Autodesk Inventor part; units mm, degrees
ref_plane "YZ Plane" through (0, 0, 0) normal (1, 0, 0) x (0, 1, 0)
ref_plane "XZ Plane" through (0, 0, 0) normal (0, 1, 0) x (-1, 0, 0)
ref_plane "XY Plane" through (0, 0, 0) normal (0, 0, 1) x (1, 0, 0)
sketch "Sketch1" plane through (0, 0, 0) normal (0, 1, 0) x (-1, 0, 0)
  circle A0 centre (0, 0) radius 14
  circle A1 centre (0, 0) radius 14
  dimension "d0" = 28
extrude "Extrusion1" add sketch "Sketch1" along normal blind 1
sketch "Sketch2" plane through (0, 1, 0) normal (0, 1, 0) x (1, 0, 0)
  circle A0 centre (0, 0) radius 13.25
  dimension "d4" = 26.5
extrude "Extrusion2" add sketch "Sketch2" along normal blind 3
sketch "Sketch3" plane through (0, 4, 0) normal (0, 1, 0) x (1, 0, 0)
  circle A0 centre (0, 0) radius 14
  dimension "d7" = 28
extrude "Extrusion3" add sketch "Sketch3" along normal blind 1
sketch "Sketch4" plane through (0, 5, 0) normal (0, 1, 0) x (1, 0, 0)
  circle A0 centre (0, 0) radius 1.25
  dimension "d10" = 2.5
hole "Hole1" at (0, 5, 0) direction (0, -1, 0) diameter 2.5 end through all
equation "\"d16\" = Thickness"
equation "\"BendRadius\" = Thickness"
equation "\"BendReliefWidth\" = Thickness"
equation "\"BendReliefDepth\" = 0.5 * Thickness"
equation "\"CornerReliefSize\" = 4 * Thickness"
equation "\"MinimumRemnant\" = 2 * Thickness"
equation "\"TransitionRadius\" = BendRadius"
equation "\"JacobiRadiusSize\" = BendRadius"
equation "\"GapSize\" = Thickness"
properties part number "wheeltemplate"
Source: CAD feature listing. Evaluate the final solid. Frame: model axes, mm. A direction names the side the tool comes from. Round coordinates to 2 decimals unless told otherwise and drop trailing zeros. Loops run counter-clockwise (first coordinate to the right, second up) from the corner with the lowest first, then second, coordinate; pieces in that order, holes last. Notation, with made-up numbers: (-31, 66.25) - (3, 66.25) arc R20 cw to (3, 79.25) - close; hole circle Ø8 at (9, -16.5). An arc over 180 degrees is marked (long way). Write item = value, one per line. Start each with the question number.
(1) Section query B-B, the plane z = 0. Output: boundary loops of the cut face in (x, y), plus the area to 3 significant figures.
(2) Section query D-D, the plane x = 11.5. Output: boundary loops of the cut face in (y, z), plus the area to 3 significant figures.
(3) Pin query (flat end, axial travel): pin 1 (1.5 mm diameter, centred on y = 3, z = -1, fed in from +X). Return the tip coordinate at first contact, or that it passes through.
(4) Ray query, line 1 along Z through (x, y) = (0, 1.3); line 2 along X through (y, z) = (4.4, -1). Return the intervals inside material, ascending. Write a range as from..to.
(5) Set-up query: faces 1 (the face through (-12.932, 0.493, 5.362)), 2 (the face through (-12.4, 1, -5.1)). Return all of +Z, -Z, +X, -X, +Y, -Y with unobstructed straight access to the full face (end or side cutting, diameter ignored); none if empty.
(6) Section query A-A, the plane x = 0. Output: boundary loops of the cut face in (y, z), plus the area to 3 significant figures.
(7) Section query C-C, the plane y = 2.15. Output: boundary loops of the cut face in (x, z).
(8) Pull-direction query (Y, two-part tool) for faces 3 (the face through (12.932, 4.493, -5.362)), 4 (the face through (0, 5, 3)), 5 (the face through (12.4, 4, 5.1)), 6 (the face through (0, 0, -3)); classes: +Y half, -Y half, draft (parallel to the pull), parting line (faces both ways), or undercut.
Conclusion:
q1.outline = (-14, 0) - (-1.25, 0) - (-1.25, 5) - (-14, 5) - (-14, 4) - (-13.25, 4) - (-13.25, 1) - (-14, 1) - close; (1.25, 0) - (14, 0) - (14, 1) - (13.25, 1) - (13.25, 4) - (14, 4) - (14, 5) - (1.25, 5) - close
q1.area = 123 mm2
q2.outline = (0, -7.98) - (1, -7.98) - (1, -6.58) - (4, -6.58) - (4, -7.98) - (5, -7.98) - (5, 7.98) - (4, 7.98) - (4, 6.58) - (1, 6.58) - (1, 7.98) - (0, 7.98) - close
q2.area = 71.4 mm2
q3.pin_1 = 13.25
q4.line_1 = -13.25..-1.25, 1.25..13.25
q4.line_2 = -13.96..-0.75, 0.75..13.96
q5.face_1 = +Y, -Y
q5.face_2 = none
q6.outline = (0, -14) - (1, -14) - (1, -13.25) - (4, -13.25) - (4, -14) - (5, -14) - (5, -1.25) - (0, -1.25) - close; (0, 1.25) - (5, 1.25) - (5, 14) - (4, 14) - (4, 13.25) - (1, 13.25) - (1, 14) - (0, 14) - close
q6.area = 123 mm2
q7.outline = circle Ø26.5 at (0, 0); hole circle Ø2.5 at (0, 0)
q8.face_3 = draft
q8.face_4 = +Y half
q8.face_5 = undercut
q8.face_6 = -Y half
